```python
from build123d import *

# Parameters (mm, degrees)
EXTRUDE_1_DEPTH     = 10
SKETCH_2_W          = 10
SKETCH_2_H          = 10
SKETCH_2_W_2        = 6.5
SKETCH_2_H_2        = 6.5
EXTRUDE_2_DEPTH     = 10
EXTRUDE_START       = 10
SKETCH_2_3_W        = 6.5
SKETCH_2_3_H        = 6.5
EXTRUDE_3_DEPTH     = 50
CUT_EXTRUDE_1_DEPTH = 80.945543966


with BuildPart() as part:
    # 草图1 → 凸台-拉伸1 (new body)
    with BuildSketch(Plane.XY):
        Polygon((0, 12.65), (0, -12.65), (40, -12.65), (40, -18.65), (-10, -18.65), (-10, 18.65), (40, 18.65), (40, 12.65), align=None)
    extrude(amount=EXTRUDE_1_DEPTH)

    # 草图2 → 凸台-拉伸2 (add)
    # profile 1 of 2: a face of its own
    with BuildSketch(Plane.ZY.offset(10)):
        with Locations((5, 0)):
            Rectangle(SKETCH_2_W, SKETCH_2_H)
        with Locations((5, 0)):
            Rectangle(SKETCH_2_W_2, SKETCH_2_H_2, mode=Mode.SUBTRACT)
    # profile 2 of 2: a face of its own
    with BuildSketch(Plane.ZY.offset(10)):
        with Locations((5, 0)):
            Rectangle(SKETCH_2_W_2, SKETCH_2_H_2)
    extrude(amount=EXTRUDE_2_DEPTH)

    # 草图2<3> → 凸台-拉伸3 (add)
    with BuildSketch(Plane.ZY.offset(10).offset(EXTRUDE_START)):
        with Locations((5, 0)):
            Rectangle(SKETCH_2_3_W, SKETCH_2_3_H)
    extrude(amount=EXTRUDE_3_DEPTH)

    # 草图3 → 切除-拉伸1 (cut, through all)
    with BuildSketch(Plane(origin=(0, 18.65, 0), x_dir=(1, 0, 0), z_dir=(0, 1, 0))):
        with BuildLine():
            ThreePointArc((32.35, -5), (35, -7.65), (37.65, -5))
            Line((37.65, -5), (32.35, -5))
        make_face()
        with BuildLine():
            Line((32.35, -5), (37.65, -5))
            ThreePointArc((37.65, -5), (35, -2.35), (32.35, -5))
        make_face()
        with BuildLine():
            ThreePointArc((35, 0), (38.535533906, -1.464466094), (40, -5))
            Line((40, -5), (40, 0))
            Line((40, 0), (35, 0))
        make_face()
        with BuildLine():
            Line((40, -10), (40, -5))
            ThreePointArc((40, -5), (38.535533906, -8.535533906), (35, -10))
            Line((35, -10), (40, -10))
        make_face()
    extrude(amount=-CUT_EXTRUDE_1_DEPTH, mode=Mode.SUBTRACT)


solid = part.part
```
Geometry: final body of the model. Coordinates: model frame, mm. A direction names the side the tool comes from. Round coordinates to 2 decimals unless told otherwise and drop trailing zeros. Order: outer loops, then holes, each group sorted by start corner. A loop starts at its lowest first (then second) coordinate and runs counter-clockwise, first axis right, second up. Notation, with made-up numbers: (60.5, 89.25) - (100.5, 89.25) arc R30 ccw to (100.5, 126.25) - close; hole circle Ø5 at (87.25, -7.75). An arc over 180 degrees is marked (long way). Use CSV: the item, a comma, the result in double quotes. Start each with the question number.
Q1. Mould query, pull axis X, two halves, no side actions, for faces 6 (the face through (32.353, 15.692, 4.883)), 7 (the face through (15, 18.65, 5)), 8 (the face through (0, 0, 5)), 9 (the face through (-10, -12, 5)). Classes: +X half, -X half, draft (parallel to the pull), parting line (faces both ways), or undercut.
Q2. Material intervals for line 1 along Y through (x, z) = (28.5, 7.5); line 2 along Z through (x, y) = (35, -14); line 3 along X through (y, z) = (16.6, 5), sorted ascending. Write a range as from..to.
Q3. Section query C-C (y = -8). Return loops of the section in (x, z).
Q4. Section query A-A (x = 15.5). Return loops of the section in (y, z).
Q5. Access query for faces 1 (the face through (-15, -5, 5)), 2 (the face through (-45, 0, 1.75)), 3 (the face through (-45, 0, 8.25)), 4 (the face through (20, 12.65, 5)), 5 (the face through (-15, 5, 5)). Directions: +Z, -Z, +X, -X, +Y, -Y. A direction counts if a zero-diameter tool reaches every point of the face in a straight line with its end or side. Return the directions, or none.
Q6. First-contact query: pin 1 (3 mm diameter, centred on x = -56, y = 1, fed in from +Z); pin 2 (6 mm diameter, centred on y = -10.5, z = 7, fed in from -X); pin 3 (3 mm diameter, centred on x = -16.5, z = 3, fed in from +Y); pin 4 (6 mm diameter, centred on y = 11, z = 6.5, fed in from +X). Flat tips, straight axial feed; report the tip coordinate or a pass-through.
Q7. Section query B-B (x = -41). Return loops of the section in (y, z).
Result set:
1,face 6,"undercut"
1,face 7,"draft"
1,face 8,"+X half"
1,face 9,"-X half"
2,line 1,"y = -18.65..-12.65, 12.65..18.65"
2,line 2,"z = 0..2.35, 7.65..10"
2,line 3,"x = -10..32.35, 37.65..40"
3,outline,"(-10, 0) - (0, 0) - (0, 10) - (-10, 10) - close"
4,outline,"(-18.65, 0) - (-12.65, 0) - (-12.65, 10) - (-18.65, 10) - close; (12.65, 0) - (18.65, 0) - (18.65, 10) - (12.65, 10) - close"
5,face 1,"+Z, -Z, -X, -Y"
5,face 2,"-Z, -X, +Y, -Y"
5,face 3,"+Z, -X, +Y, -Y"
5,face 4,"+Z, -Z, +X"
5,face 5,"+Z, -Z, -X, +Y"
6,pin 1,"stops at z = 8.25"
6,pin 2,"stops at x = -10"
6,pin 3,"stops at y = 5"
6,pin 4,"stops at x = 40"
7,outline,"(-3.25, 1.75) - (3.25, 1.75) - (3.25, 8.25) - (-3.25, 8.25) - close"
